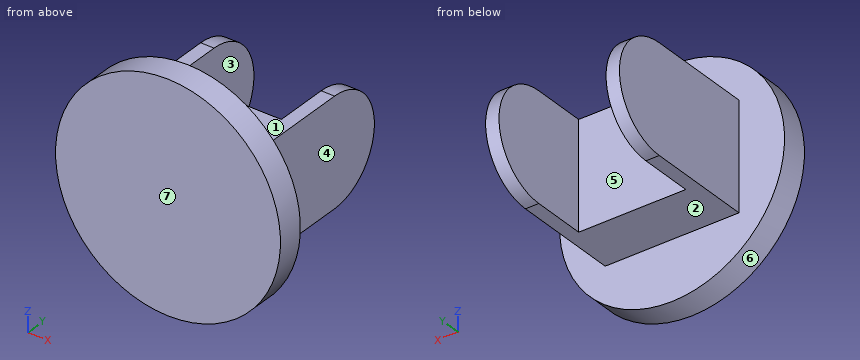
from build123d import *

# Parameters (mm, degrees)
BOSS_EXTRUDE1_DEPTH = 100
SKETCH2_R           = 84.031242374
BOSS_EXTRUDE2_DEPTH = 20
SKETCH3_W           = 80
SKETCH3_H           = 80
CUT_EXTRUDE1_DEPTH  = 200.369313128


with BuildPart() as part:
    # Sketch1 → Boss-Extrude1 (new body)
    with BuildSketch(Plane(origin=(0, 0, 0), x_dir=(0, 0, -1), z_dir=(1, 0, 0))):
        with BuildLine():
            Line((-40, 40), (-40, -40))
            Line((-40, -40), (40, -40))
            Line((40, -40), (40, 40))
            ThreePointArc((40, 40), (0, 80), (-40, 40))
        make_face()
    extrude(amount=BOSS_EXTRUDE1_DEPTH)

    # Sketch2 → Boss-Extrude2 (add)
    with BuildSketch(Plane.XZ.offset(40)):
        with Locations(Location((50, 0, 0), (0, 0, 270))):
            Circle(SKETCH2_R)
    extrude(amount=BOSS_EXTRUDE2_DEPTH)

    # Sketch3 → Cut-Extrude1 (cut, through all)
    with BuildSketch(Plane.XY.offset(40)):
        with Locations((50, 40)):
            Rectangle(SKETCH3_W, SKETCH3_H)
    extrude(amount=-CUT_EXTRUDE1_DEPTH, mode=Mode.SUBTRACT)


solid = part.part
Geometry: final body of the model. Coordinates: model frame, mm. Face numbers are marked on the shaded views. A direction names the side the tool comes from. Give positions to 0.01 mm unless a question says otherwise; leave off trailing zeros. Write each loop counter-clockwise with the first axis right and the second up, starting at its lowest first coordinate (ties: lowest second). Pieces come first, ordered by that corner, then holes. Notation, with made-up numbers: (-30.75, 34.5) -> (-6.75, 34.5) arc R9 ccw to (-6.75, 38.5) -> close; hole circle Ø11 at (47, 26.25). An arc over 180 degrees is marked (long way). Answer in a Markdown table with one row per item.
(1) Pin query (flat end, axial travel): pin 1 (8 mm diameter, centred on y = 19, z = 43, fed in from -X); pin 2 (8 mm diameter, centred on x = 82.5, y = 12, fed in from -Z); pin 3 (5 mm diameter, centred on y = -45, z = -13.5, fed in from -X); pin 4 (1 mm diameter, centred on y = -42.5, z = -3.5, fed in from -X). Return the tip coordinate at first contact, or that it passes through.
Answers below:
| item | result |
|---|---|
| pin 1 | x = 0 |
| pin 2 | through |
| pin 3 | x = -33.31 |
| pin 4 | x = -33.98 |
(2) Set-up query: the marked faces 1, 2, 3 and 4. Return all of +Z, -Z, +X, -X, +Y, -Y with unobstructed straight access to the full face (end or side cutting, diameter ignored); none if empty.
Answers below:
| item | result |
|---|---|
| face 1 | +Z, +X, -X, +Y |
| face 2 | -Z, +X, -X, +Y |
| face 3 | +Z, -Z, +Y |
| face 4 | +Z, -Z, +X, +Y |
(3) Ray query, line 1 along X through (y, z) = (65.5, 21.5); line 2 along Z through (x, y) = (10, -3.5); line 3 along Y through (x, z) = (44, 53.5). Return the intervals inside material, ascending. Write a range as [from, to].
Answers below:
| item | result |
|---|---|
| line 1 | [0, 10], [90, 100] |
| line 2 | [-40, 40] |
| line 3 | [-60, -40] |
(4) Section query D-D on y = -4.5. Return loops of the section in (x, z), then the cut area to 3 significant figures.
Answers below:
| item | result |
|---|---|
| outline | (0, -40) -> (100, -40) -> (100, 40) -> (0, 40) -> close |
| area | 8,000 mm^2 |
(5) Section query A-A on y = 23.5. Return loops of the section in (x, z), then the cut area to 3 significant figures.
Answers below:
| item | result |
|---|---|
| outline | (0, -40) -> (10, -40) -> (10, 40) -> (0, 40) -> close; (90, -40) -> (100, -40) -> (100, 40) -> (90, 40) -> close |
| area | 1,600 mm^2 |
(6) Section query C-C on x = 50. Return loops of the section in (y, z).
Answers below:
| item | result |
|---|---|
| outline | (-60, -84.03) -> (-40, -84.03) -> (-40, -40) -> (0, -40) -> (0, 40) -> (-40, 40) -> (-40, 84.03) -> (-60, 84.03) -> close |
(7) Draft query along X for the marked faces 5, 6 and 7. Return one class per face: +X half, -X half, draft (parallel to the pull), parting line (faces both ways), or undercut.
Answers below:
| item | result |
|---|---|
| face 5 | undercut |
| face 6 | parting line |
| face 7 | draft |
(8) Section query B-B on z = 0. Return loops of the section in (x, y).
Answers below:
| item | result |
|---|---|
| outline | (-34.03, -60) -> (134.03, -60) -> (134.03, -40) -> (100, -40) -> (100, 80) -> (90, 80) -> (90, 0) -> (10, 0) -> (10, 80) -> (0, 80) -> (0, -40) -> (-34.03, -40) -> close |
